from build123d import *

# Parameters (mm, degrees)
SKETCH2_R                    = 6
BOSS_EXTRUDE1_DEPTH          = 6
BOSS_EXTRUDE2_DEPTH          = 30
CUT_EXTRUDE1_DEPTH           = 47.38051854
CUT_EXTRUDE1_DEPTH_BACK      = 47.38051854
SKETCH3_R                    = 1.7
SKETCH4_R                    = 2.75
CUT_EXTRUDE2_DEPTH           = 2
CUT_EXTRUDE2_OTHER_WAY_DEPTH = 10
CUT_EXTRUDE2_OTHER_WAY_TAPER = -11
CUT_EXTRUDE3_DEPTH           = 45.727983411
CUT_EXTRUDE3_DEPTH_BACK      = 45.727983411
SKETCH6_R                    = 1.75
SKETCH7_R                    = 3.25
CUT_EXTRUDE4_DEPTH           = 2


with BuildPart() as part:
    # Sketch2 → Boss-Extrude1 (new body)
    with BuildSketch(Plane(origin=(0, 0, 0), x_dir=(1, 0, 0), z_dir=(0, 1, 0))):
        Polygon((-6.162811814, 16.2), (-9.922811814, 11.5), (-19.51, 11.5), (-19.51, -1.421485233), (-20.95, -3.221485233), (-20.95, -16.3), (-6.037188186, -16.3), (-4.837188186, -14.8), (4.837188186, -14.8), (6.037188186, -16.3), (20.95, -16.3), (20.95, -3.221485233), (19.51, -1.421485233), (19.51, 11.5), (9.922811814, 11.5), (6.162811814, 16.2), align=None)
        with Locations(Location((0, 0, 0), (0, 0, 270))):
            Circle(SKETCH2_R, mode=Mode.SUBTRACT)
    extrude(amount=BOSS_EXTRUDE1_DEPTH)

    # Sketch2<3> → Boss-Extrude2 (add)
    with BuildSketch(Plane(origin=(0, 0, 0), x_dir=(1, 0, 0), z_dir=(0, 1, 0))):
        Polygon((9.922811814, 11.5), (6.162811814, 16.2), (-6.162811814, 16.2), (-9.922811814, 11.5), (-19.51, 11.5), (-19.51, -1.421485233), (-20.95, -3.221485233), (-20.95, -16.3), (-6.037188186, -16.3), (-4.837188186, -14.8), (4.837188186, -14.8), (6.037188186, -16.3), (20.95, -16.3), (20.95, -3.221485233), (19.51, -1.421485233), (19.51, 11.5), align=None)
        Polygon((4.240312424, 12.2), (-4.240312424, 12.2), (-8.000312424, 7.5), (-15.51, 7.5), (-15.51, -2.82460947), (-16.95, -4.62460947), (-16.95, -12.3), (-7.959687576, -12.3), (-6.759687576, -10.8), (6.759687576, -10.8), (7.959687576, -12.3), (16.95, -12.3), (16.95, -4.62460947), (15.51, -2.82460947), (15.51, 7.5), (8.000312424, 7.5), align=None, mode=Mode.SUBTRACT)
    extrude(amount=-BOSS_EXTRUDE2_DEPTH)

    # Sketch3 → Cut-Extrude1 (cut, two sides: drawn at the far end of the back side and taken through both)
    with BuildSketch(Plane(origin=(0, 0, 12.3), x_dir=(-1, 0, 0), z_dir=(0, 0, -1)).offset(-CUT_EXTRUDE1_DEPTH_BACK)):
        with Locations((10.9, -5.2)):
            Circle(SKETCH3_R)
        with Locations((10.9, -24)):
            Circle(SKETCH3_R)
        with Locations((-11.8, -23.7)):
            Circle(SKETCH3_R)
        with Locations((-11.8, -5.1)):
            Circle(SKETCH3_R)
    extrude(amount=CUT_EXTRUDE1_DEPTH + CUT_EXTRUDE1_DEPTH_BACK, mode=Mode.SUBTRACT)

    # Sketch4 → Cut-Extrude2 (cut)
    with BuildSketch(Plane(origin=(0, 0, -11.5), x_dir=(-1, 0, 0), z_dir=(0, 0, -1))):
        with Locations((-11.8, -5.1)):
            Circle(SKETCH4_R)
        with Locations((10.9, -5.2)):
            Circle(SKETCH4_R)
        with Locations((-11.8, -23.7)):
            Circle(SKETCH4_R)
        with Locations((10.9, -24)):
            Circle(SKETCH4_R)
    extrude(amount=-CUT_EXTRUDE2_DEPTH, mode=Mode.SUBTRACT)

    # Sketch4 → Cut-Extrude2 other way (cut)
    with BuildSketch(Plane(origin=(0, 0, -11.5), x_dir=(-1, 0, 0), z_dir=(0, 0, -1))):
        with Locations((-11.8, -5.1)):
            Circle(SKETCH4_R)
        with Locations((10.9, -5.2)):
            Circle(SKETCH4_R)
        with Locations((-11.8, -23.7)):
            Circle(SKETCH4_R)
        with Locations((10.9, -24)):
            Circle(SKETCH4_R)
    extrude(amount=CUT_EXTRUDE2_OTHER_WAY_DEPTH, taper=CUT_EXTRUDE2_OTHER_WAY_TAPER, mode=Mode.SUBTRACT)

    # Sketch6 → Cut-Extrude3 (cut, two sides: drawn at the far end of the back side and taken through both)
    with BuildSketch(Plane(origin=(0, 6, 0), x_dir=(1, 0, 0), z_dir=(0, 1, 0)).offset(-CUT_EXTRUDE3_DEPTH_BACK)):
        with Locations(Location((-12, -4.25, 0), (0, 0, 270))):
            Circle(SKETCH6_R)
        with Locations(Location((12, -4.25, 0), (0, 0, 270))):
            Circle(SKETCH6_R)
    extrude(amount=CUT_EXTRUDE3_DEPTH + CUT_EXTRUDE3_DEPTH_BACK, mode=Mode.SUBTRACT)

    # Sketch7 → Cut-Extrude4 (cut)
    with BuildSketch(Plane.XZ):
        with Locations(Location((-12, 4.25, 0), (0, 0, 270))):
            Circle(SKETCH7_R)
        with Locations(Location((12, 4.25, 0), (0, 0, 270))):
            Circle(SKETCH7_R)
    extrude(amount=-CUT_EXTRUDE4_DEPTH, mode=Mode.SUBTRACT)


solid = part.part
Check sheet for the modelled part. Datum: model origin and axes. Units: mm. A direction names the side the tool comes from. Round coordinates to 2 decimals unless told otherwise and drop trailing zeros. Loops run counter-clockwise (first coordinate to the right, second up) from the corner with the lowest first, then second, coordinate; pieces in that order, holes last. Notation, with made-up numbers: M -2,29.5 L 24,29.5 A24 ccw 24,44.5 Z; hole C -6.5,-35 d5. An arc over 180 degrees is marked long. One line per question, with ' | ' between items. Start each with the question number.
Item 1: Gauge pin test, flat ends, axial feed: pin 1 Ø4.5 at (x, y) = (-14, -20) entering from -Z; pin 2 Ø19 at (x, z) = (0, 0) entering from -Y; pin 3 Ø6 at (x, z) = (-12, 4.25) entering from -Y; pin 4 Ø4 at (x, z) = (12, 4.25) entering from +Y. Record the tip position at first contact, or that the pin passes through.
Item 2: Scan lines: probe 1 along X at (y, z) = (-5, -10); probe 2 along Y at (x, z) = (11.8, 15.4); probe 3 along X at (y, z) = (4.8, 4.25). Record each from-to range of solid material in increasing order.
Item 3: Section check C-C (x = 3). Record the boundary of the cut face in (y, z), and give its area (3 significant figures).
Item 4: Section check B-B (z = 10). Record the boundary of the cut face in (x, y), and give its area (3 significant figures).
Item 5: Release check for a two-part mould opening along X. For faces 1 (the face through (20.24, -11.748, 2.334)), 2 (the face through (0, -12, -16.2)), 3 (the face through (15, 1, 3)), 4 (the face through (-8.02, -11.75, -13.88)) record: released by +X, released by -X, zero draft, split by the parting line, or undercut.
Item 6: Set-up check for faces 5 (the face through (16.95, -15, 9)), 6 (the face through (19.51, -12, -5)), 7 (the face through (-13, -5, -9.5)): record each of +Z, -Z, +X, -X, +Y, -Y from which the full face is reachable in a straight line by a thin tool's end or side.
Worked out:
1) pin 1: z = -11.5 | pin 2: y = 0 | pin 3: y = 2 | pin 4: y = 6
2) probe 1: -19.51 to -13.64, -8.16 to -6, 6 to 9.05, 14.55 to 19.51 | probe 2: -30 to -25.4, -22 to -6.8, -3.4 to 6 | probe 3: -20.95 to -13.75, -10.25 to -4.24, 4.24 to 10.25, 13.75 to 20.95
3) outline: M -30,-16.2 L 6,-16.2 L 6,-5.2 L 0,-5.2 L 0,-12.2 L -30,-12.2 Z; M -30,10.8 L 0,10.8 L 0,5.2 L 6,5.2 L 6,14.8 L -30,14.8 Z | area: 364 mm^2
4) outline: M -20.95,-30 L -16.95,-30 L -16.95,0 L 16.95,0 L 16.95,-30 L 20.95,-30 L 20.95,6 L -20.95,6 Z | area: 491 mm^2
5) face 1: released by +X | face 2: zero draft | face 3: undercut | face 4: released by -X
6) face 5: -Y | face 6: -Z, +X, +Y, -Y | face 7: -Z
